Part model, mm, in its own coordinate system. Face numbers are marked on the shaded views. A direction names the side the tool comes from. Give positions to 0.01 mm unless a question says otherwise; leave off trailing zeros. Order: outer loops, then holes, each group sorted by start corner. A loop starts at its lowest first (then second) coordinate and runs counter-clockwise, first axis right, second up. Notation, with made-up numbers: M 56.5,-11.75 L 60.5,-11.75 A9 ccw 60.5,5.25 Z; hole C 31.25,17.25 d3. An arc over 180 degrees is marked long. Answer as a JSON object with one key per item and string values.
from build123d import *

# Parameters (mm, degrees)
ESQUISSE1_R                  = 10.5
BOSS_EXTRU_1_DEPTH           = 10
ESQUISSE2_R                  = 8
BOSS_EXTRU_2_DEPTH           = 16
ESQUISSE3_W                  = 2
ESQUISSE3_H                  = 16
ENL_V_MAT_EXTRU_1_DEPTH      = 14
CHANFREIN1_SIZE              = 1
ENL_V_MAT_EXTRU_2_DEPTH      = 33.53459697
ENL_V_MAT_EXTRU_2_DEPTH_BACK = 33.53459697
ESQUISSE4_R                  = 3
BOSS_EXTRU_3_START           = 85
ESQUISSE5_R                  = 8
BOSS_EXTRU_3_DEPTH           = 85
ESQUISSE6_R                  = 10.5
BOSS_EXTRU_4_DEPTH           = 10
BOSS_EXTRU_5_START           = 16
ESQUISSE7_R                  = 8
BOSS_EXTRU_5_DEPTH           = 16
ESQUISSE8_R                  = 3
ENL_V_MAT_EXTRU_3_DEPTH      = 98


with BuildPart() as part:
    # Esquisse1 → Boss.-Extru.1 (new body)
    with BuildSketch(Plane.XY):
        Circle(ESQUISSE1_R)
    extrude(amount=BOSS_EXTRU_1_DEPTH)

    # Esquisse2 → Boss.-Extru.2 (add)
    with BuildSketch(Plane.XY.offset(10)):
        Circle(ESQUISSE2_R)
    extrude(amount=BOSS_EXTRU_2_DEPTH)

    # Esquisse3 → Enlèv. mat.-Extru.1 (cut)
    with BuildSketch(Plane.XY.offset(26)):
        with Locations((-7, 0)):
            Rectangle(ESQUISSE3_W, ESQUISSE3_H)
        with Locations((7, 0)):
            Rectangle(ESQUISSE3_W, ESQUISSE3_H)
    extrude(amount=-ENL_V_MAT_EXTRU_1_DEPTH, mode=Mode.SUBTRACT)

    # Chanfrein1
    chanfrein1_edges = [part.edges().sort_by_distance(p)[0] for p in [
        (0, -8, 26),
        (-6, 0, 26),
        (-6, 0, 12),
        (0, 8, 26),
        (6, 0, 26),
        (6, 0, 12),
    ]]
    chamfer(chanfrein1_edges, length=CHANFREIN1_SIZE)

    # Esquisse4 → Enlèv. mat.-Extru.2 (cut, two sides: drawn at the far end of the back side and taken through both)
    with BuildSketch(Plane.ZY.offset(6).offset(-ENL_V_MAT_EXTRU_2_DEPTH_BACK)):
        with Locations((19, 0)):
            Circle(ESQUISSE4_R)
    extrude(amount=ENL_V_MAT_EXTRU_2_DEPTH + ENL_V_MAT_EXTRU_2_DEPTH_BACK, mode=Mode.SUBTRACT)

    # Esquisse5 → Boss.-Extru.3 (add)
    with BuildSketch(Plane(origin=(0, 0, 0), x_dir=(-1, 0, 0), z_dir=(0, 0, -1)).offset(BOSS_EXTRU_3_START)):
        with Locations(Location((0, 0, 0), (0, 0, 28.955024372))):
            Circle(ESQUISSE5_R)
    extrude(amount=-BOSS_EXTRU_3_DEPTH)

    # Esquisse6 → Boss.-Extru.4 (add)
    with BuildSketch(Plane(origin=(0, 0, -85), x_dir=(-1, 0, 0), z_dir=(0, 0, -1))):
        with Locations(Location((0, 0, 0), (0, 0, 180))):
            Circle(ESQUISSE6_R)
    extrude(amount=-BOSS_EXTRU_4_DEPTH)

    # Esquisse7 → Boss.-Extru.5 (add)
    with BuildSketch(Plane(origin=(0, 0, -85), x_dir=(-1, 0, 0), z_dir=(0, 0, -1)).offset(BOSS_EXTRU_5_START)):
        with Locations(Location((0, 0, 0), (0, 0, 180))):
            Circle(ESQUISSE7_R)
    extrude(amount=-BOSS_EXTRU_5_DEPTH)

    # Esquisse8 → Enlèv. mat.-Extru.3 (cut)
    with BuildSketch(Plane(origin=(0, 0, -101), x_dir=(-1, 0, 0), z_dir=(0, 0, -1))):
        Circle(ESQUISSE8_R)
    extrude(amount=-ENL_V_MAT_EXTRU_3_DEPTH, mode=Mode.SUBTRACT)


solid = part.part
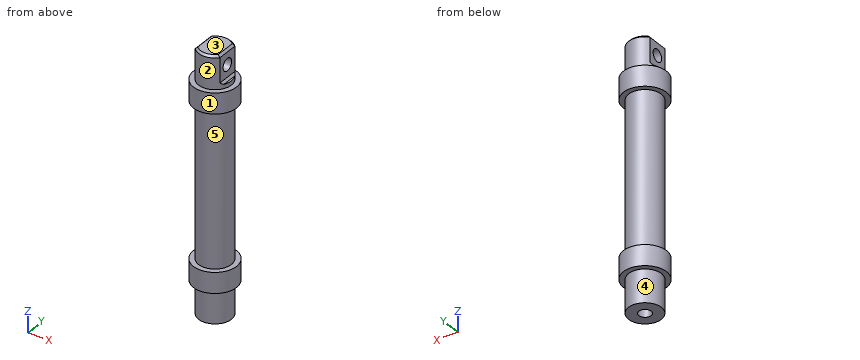
1. Cut at C-C on z = -61.5. Give the cut face in (x, y), plus the area to 3 significant figures.
Worked answers:
{"outline": "C 0,0 d16; hole C 0,0 d6", "area": "173 mm^2"}
2. Probe line 1 along Z through (x, y) = (6, -7); line 2 along Y through (x, z) = (0, -62); line 3 along Z through (x, y) = (-3.5, 0). List the from-to ranges inside material, lowest first.
Worked answers:
{"line 1": "z = -85 to -75, 0 to 10", "line 2": "y = -8 to -3, 3 to 8", "line 3": "z = -101 to 16, 22 to 26"}
3. Two-plate mould, pull along Z, no slides. Class the marked faces 3, 4 and 5: +Z half, -Z half, draft (parallel to the pull), parting line (faces both ways), or undercut.
Worked answers:
{"face 3": "+Z half", "face 4": "draft", "face 5": "undercut"}
4. Which spindle directions (+Z, -Z, +X, -X, +Y, -Y) get a long thin tool onto all of the face, cutting with end or side? Do the marked faces 1 and 2. Say none if no direction does.
Worked answers:
{"face 1": "+Z, -Z", "face 2": "+Z"}
5. Cut at A-A on z = 19. Give the cut face in (x, y), plus the area to 3 significant figures.
Worked answers:
{"outline": "M -6,-5.29 A8 ccw 6,-5.29 L 6,-3 L -6,-3 Z; M -6,3 L 6,3 L 6,5.29 A8 ccw -6,5.29 Z", "area": "100 mm^2"}
6. Cut at B-B on x = 0. Give the cut face in (y, z), plus the area to 3 significant figures.
Worked answers:
{"outline": "M -10.5,-85 L -8,-85 L -8,-101 L -3,-101 L -3,-3 L 3,-3 L 3,-101 L 8,-101 L 8,-85 L 10.5,-85 L 10.5,-75 L 8,-75 L 8,0 L 10.5,0 L 10.5,10 L 8,10 L 8,25 L 7,26 L -7,26 L -8,25 L -8,10 L -10.5,10 L -10.5,0 L -8,0 L -8,-75 L -10.5,-75 Z; hole C 0,19 d6", "area": "1,510 mm^2"}
7. Pin check, flat tips, straight feed: P1, Ø8.5, axis at y = 2, z = 16.5, coming from the -X side; P2, Ø2, axis at x = 0.5, z = -46.5, coming from the +Y side; P3, Ø7, axis at y = 0, z = 19, coming from the +X side. Stop position of each tip, or through.
Worked answers:
{"P1": "stops at x = -6.75", "P2": "stops at y = 8", "P3": "stops at x = 6"}
